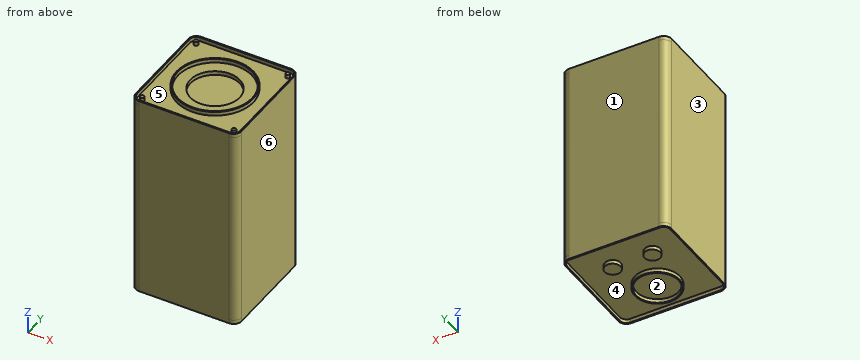
```python
from build123d import *

# Parameters (mm, degrees)
SKETCH_2_W          = 80
SKETCH_2_H          = 80
EXTRUDE_1_DEPTH     = 150
FILLET_1_R          = 6
EXTRUDE_START       = 3
EXTRUDE_2_DEPTH     = 3
EXTRUDE_5_DEPTH     = 3
SKETCH_7_R          = 17
SKETCH_7_R_2        = 16
SKETCH_7_R_3        = 5.982349016
EXTRUDE_6_DEPTH     = 3
SKETCH_8_R          = 29
SKETCH_8_R_2        = 28
EXTRUDE_7_DEPTH     = 3
SKETCH_9_R          = 1.5
EXTRUDE_8_DEPTH     = 3
SKETCH_10_R         = 18.744403632
CUT_EXTRUDE_1_DEPTH = 3


with BuildPart() as part:
    # 草图2 → 凸台-拉伸1 (new body)
    with BuildSketch(Plane.XY):
        Rectangle(SKETCH_2_W, SKETCH_2_H)
    extrude(amount=EXTRUDE_1_DEPTH)

    # 圆角1
    fillet_1_edges = [part.edges().sort_by_distance(p)[0] for p in [
        (40, -40, 75),
        (-40, -40, 75),
        (-40, 40, 75),
        (40, 40, 75),
    ]]
    fillet(fillet_1_edges, radius=FILLET_1_R)

    # 草图3 → 凸台-拉伸2 (add)
    with BuildSketch(Plane.XY.offset(150).offset(EXTRUDE_START)):
        with BuildLine():
            Line((-40, 34), (-40, -34))
            ThreePointArc((-40, -34), (-38.242640687, -38.242640687), (-34, -40))
            Line((-34, -40), (34, -40))
            ThreePointArc((34, -40), (38.242640687, -38.242640687), (40, -34))
            Line((40, -34), (40, 34))
            ThreePointArc((40, 34), (38.242640687, 38.242640687), (34, 40))
            Line((34, 40), (-34, 40))
            ThreePointArc((-34, 40), (-38.242640687, 38.242640687), (-40, 34))
        make_face()
        with BuildLine():
            Line((34, 39), (-34, 39))
            ThreePointArc((-34, 39), (-37.535533906, 37.535533906), (-39, 34))
            Line((-39, 34), (-39, -34))
            ThreePointArc((-39, -34), (-37.535533906, -37.535533906), (-34, -39))
            Line((-34, -39), (34, -39))
            ThreePointArc((34, -39), (37.535533906, -37.535533906), (39, -34))
            Line((39, -34), (39, 34))
            ThreePointArc((39, 34), (37.535533906, 37.535533906), (34, 39))
        make_face(mode=Mode.SUBTRACT)
    extrude(amount=-EXTRUDE_2_DEPTH)

    # 草图6 → 凸台-拉伸5 (add)
    with BuildSketch(Plane(origin=(0, 0, 0), x_dir=(-1, 0, 0), z_dir=(0, 0, -1))):
        with BuildLine():
            Line((-34, -40), (34, -40))
            ThreePointArc((34, -40), (38.242640687, -38.242640687), (40, -34))
            Line((40, -34), (40, 34))
            ThreePointArc((40, 34), (38.242640687, 38.242640687), (34, 40))
            Line((34, 40), (-34, 40))
            ThreePointArc((-34, 40), (-38.242640687, 38.242640687), (-40, 34))
            Line((-40, 34), (-40, -34))
            ThreePointArc((-40, -34), (-38.242640687, -38.242640687), (-34, -40))
        make_face()
        with BuildLine():
            Line((34, 39), (-34, 39))
            ThreePointArc((-34, 39), (-37.535533906, 37.535533906), (-39, 34))
            Line((-39, 34), (-39, -34))
            ThreePointArc((-39, -34), (-37.535533906, -37.535533906), (-34, -39))
            Line((-34, -39), (34, -39))
            ThreePointArc((34, -39), (37.535533906, -37.535533906), (39, -34))
            Line((39, -34), (39, 34))
            ThreePointArc((39, 34), (37.535533906, 37.535533906), (34, 39))
        make_face(mode=Mode.SUBTRACT)
    extrude(amount=EXTRUDE_5_DEPTH)

    # 草图7 → 凸台-拉伸6 (add)
    # profile 1 of 3: a face of its own
    with BuildSketch(Plane(origin=(0, 0, 0), x_dir=(-1, 0, 0), z_dir=(0, 0, -1))):
        with Locations((0, -16)):
            Circle(SKETCH_7_R)
        with Locations((0, -16)):
            Circle(SKETCH_7_R_2, mode=Mode.SUBTRACT)
    # profile 2 of 3: a face of its own
    with BuildSketch(Plane(origin=(0, 0, 0), x_dir=(-1, 0, 0), z_dir=(0, 0, -1))):
        with Locations((15, 16)):
            Circle(SKETCH_7_R_3)
    # profile 3 of 3: a face of its own
    with BuildSketch(Plane(origin=(0, 0, 0), x_dir=(-1, 0, 0), z_dir=(0, 0, -1))):
        with Locations(Location((-15, 16, 0), (0, 0, 180))):
            Circle(SKETCH_7_R_3)
    extrude(amount=EXTRUDE_6_DEPTH)

    # 草图8 → 凸台-拉伸7 (add)
    with BuildSketch(Plane.XY.offset(150)):
        with Locations(Location((0, 0, 0), (0, 0, 180))):
            Circle(SKETCH_8_R)
        Circle(SKETCH_8_R_2, mode=Mode.SUBTRACT)
    extrude(amount=EXTRUDE_7_DEPTH)

    # 草图9 → 凸台-拉伸8 (add)
    with BuildSketch(Plane.XY.offset(150)):
        with Locations(Location((-34.649983427, 34.649983427, 0), (0, 0, 180))):
            Circle(SKETCH_9_R)
        with Locations(Location((34.649983427, 34.649983427, 0), (0, 0, 180))):
            Circle(SKETCH_9_R)
        with Locations(Location((34.649983427, -34.649983427, 0), (0, 0, 180))):
            Circle(SKETCH_9_R)
        with Locations(Location((-34.649983427, -34.649983427, 0), (0, 0, 180))):
            Circle(SKETCH_9_R)
    extrude(amount=EXTRUDE_8_DEPTH)

    # 草图10 → 切除-拉伸1 (cut)
    with BuildSketch(Plane.XY.offset(150)):
        Circle(SKETCH_10_R)
    extrude(amount=-CUT_EXTRUDE_1_DEPTH, mode=Mode.SUBTRACT)


solid = part.part
```
The listing builds one solid part. Answer for the finished solid, in the listing's coordinates (mm). Face numbers are marked on the shaded views. A direction names the side the tool comes from. Round coordinates to 2 decimals unless told otherwise and drop trailing zeros. Write each loop counter-clockwise with the first axis right and the second up, starting at its lowest first coordinate (ties: lowest second). Pieces come first, ordered by that corner, then holes. Notation, with made-up numbers: (-38.5, 16.5) -> (-15.5, 16.5) arc R13 ccw to (-15.5, 20.5) -> close; hole circle Ø10 at (19, -22.75). An arc over 180 degrees is marked (long way). Answer as a JSON object with one key per item and string values. Group by question number.
Q1. Straight lines are drawn through the part: line 1 along Y through (x, z) = (0, -2); line 2 along Y through (x, z) = (0, 152.1); line 3 along Y through (x, z) = (0, 148). For each, find the intervals that lie inside material, in ascending order.
Q2. Determine the mould class of the marked faces 1, 2 and 3 for opening direction X: pulls with the +X half, pulls with the -X half, needs draft (parallel to the pull), parting line crosses it, or undercut.
Q3. Which of the six approach directions +Z, -Z, +X, -X, +Y, -Y give full straight-line access (tool end or side, diameter ignored) to the marked faces 4, 5 and 6?
Q4. Section C-C (y = 25.5) is taken. Write down the section's boundary in (x, z), plus the area to 3 significant figures.
Q5. Each of these flat-tipped pins is pushed along its axis until it touches: pin 1 Ø5 at (x, y) = (-28, -17.5) entering from -Z; pin 2 Ø8 at (x, y) = (20.5, -3) entering from +Z. Where does it stop, or does it pass through?
Q6. Section D-D (y = -23.5) is taken. Write down the section's boundary in (x, z).
Check values:
{
 "1": {"line 1": "-40 to -39, -33 to -32, 0 to 1, 39 to 40", "line 2": "-40 to -39, -29 to -28, 28 to 29, 39 to 40", "line 3": "-40 to -18.74, 18.74 to 40"},
 "2": {"face 1": "needs draft", "face 2": "undercut", "face 3": "pulls with the -X half"},
 "3": {"face 4": "-Z", "face 5": "+Z", "face 6": "+Z, -Z, +X, +Y, -Y"},
 "4": {"outline": "(-40, -3) -> (-39, -3) -> (-39, 0) -> (39, 0) -> (39, -3) -> (40, -3) -> (40, 153) -> (39, 153) -> (39, 150) -> (13.81, 150) -> (13.81, 153) -> (11.57, 153) -> (11.57, 150) -> (-11.57, 150) -> (-11.57, 153) -> (-13.81, 153) -> (-13.81, 150) -> (-39, 150) -> (-39, 153) -> (-40, 153) -> close", "area": "12,000 mm^2"},
 "5": {"pin 1": "z = 0", "pin 2": "z = 150"},
 "6": {"outline": "(-40, -3) -> (-39, -3) -> (-39, 0) -> (-15.26, 0) -> (-15.26, -3) -> (-14.13, -3) -> (-14.13, 0) -> (14.13, 0) -> (14.13, -3) -> (15.26, -3) -> (15.26, 0) -> (39, 0) -> (39, -3) -> (40, -3) -> (40, 153) -> (39, 153) -> (39, 150) -> (16.99, 150) -> (16.99, 153) -> (15.22, 153) -> (15.22, 150) -> (-15.22, 150) -> (-15.22, 153) -> (-16.99, 153) -> (-16.99, 150) -> (-39, 150) -> (-39, 153) -> (-40, 153) -> close"}
}
